Input: part model. Units: mm. Frame: model coordinates. A direction names the side the tool comes from. Give positions to 0.01 mm unless a question says otherwise; leave off trailing zeros. Write each loop counter-clockwise with the first axis right and the second up, starting at its lowest first coordinate (ties: lowest second). Pieces come first, ordered by that corner, then holes.
```python
from build123d import *

# Parameters (mm, degrees)
SKETCH1_W                = 400
SKETCH1_H                = 200
BOSS_EXTRUDE1_DEPTH      = 600
SHELL1_T                 = -10
BOSS_EXTRUDE2_DEPTH      = 25
BOSS_EXTRUDE2_DEPTH_BACK = 10
SKETCH2_W                = 60
SKETCH2_H                = 60
SKETCH3_R                = 7.5
SKETCH3_R_2              = 5
BOSS_EXTRUDE3_DEPTH      = 15
LPATTERN1_COUNT          = 2
LPATTERN1_PITCH          = 330
LPATTERN1_COUNT_DIR2     = 2
LPATTERN1_PITCH_DIR2     = 530
SKETCH4_R                = 15
CUT_EXTRUDE1_DEPTH       = 749.331477355
BOSS_EXTRUDE4_START      = 15
SKETCH5_R                = 25
SKETCH5_R_2              = 15
BOSS_EXTRUDE4_DEPTH      = 15
THICKEN1_START           = 375
THICKEN1_OUTLINE_W       = 31
THICKEN1_OUTLINE_H       = 30
THICKEN1_DEPTH           = 0.5
THICKEN2_START           = 24.5
THICKEN2_OUTLINE_W       = 31
THICKEN2_OUTLINE_H       = 30
THICKEN2_DEPTH           = 0.5
BOSS_EXTRUDE6_REACH      = 737.941
SKETCH7_W                = 380
SKETCH7_H                = 580
SKETCH10_R               = 67.5
CUT_EXTRUDE2_DEPTH       = 60
SKETCH11_R               = 25
BOSS_EXTRUDE7_DEPTH      = 25
BOSS_EXTRUDE8_DEPTH      = 55
SKETCH11_4_R             = 15
CUT_EXTRUDE4_DEPTH       = 20


# Read off the part's stored shape, not the designer's step: Thicken1, Thicken2
with BuildPart() as part:
    # Sketch1 → Boss-Extrude1 (new body)
    with BuildSketch(Plane.XY):
        with Locations((200, 100)):
            Rectangle(SKETCH1_W, SKETCH1_H)
    extrude(amount=BOSS_EXTRUDE1_DEPTH)

    # Shell1
    shell1_openings = [part.faces().sort_by_distance(p)[0] for p in [
        (200, 0, 300),
    ]]
    offset(amount=SHELL1_T, openings=shell1_openings, kind=Kind.INTERSECTION)

    # Sketch2 → Boss-Extrude2 (add, two sides: drawn at the far end of the back side and taken through both)
    with BuildSketch(Plane(origin=(0, 28, 0), x_dir=(1, 0, 0), z_dir=(0, 1, 0)).offset(-BOSS_EXTRUDE2_DEPTH_BACK)):
        with Locations((370, -570)):
            Rectangle(SKETCH2_W, SKETCH2_H)
        with Locations((30, -570)):
            Rectangle(SKETCH2_W, SKETCH2_H)
        with Locations((370, -30)):
            Rectangle(SKETCH2_W, SKETCH2_H)
        with Locations((30, -30)):
            Rectangle(SKETCH2_W, SKETCH2_H)
    extrude(amount=BOSS_EXTRUDE2_DEPTH + BOSS_EXTRUDE2_DEPTH_BACK)

    # Sketch3 → Boss-Extrude3 (add)
    with BuildSketch(Plane(origin=(0, 18, 0), x_dir=(1, 0, 0), z_dir=(0, 1, 0))):
        with Locations(Location((35, -565, 0), (0, 0, 270))):
            Circle(SKETCH3_R)
        with Locations(Location((35, -565, 0), (0, 0, 270))):
            Circle(SKETCH3_R_2, mode=Mode.SUBTRACT)
    boss_extrude3 = extrude(amount=-BOSS_EXTRUDE3_DEPTH)

    # LPattern1: Boss-Extrude3 2 × 2
    with Locations(*[(i * LPATTERN1_PITCH, 0, -j * LPATTERN1_PITCH_DIR2) for i in range(LPATTERN1_COUNT) for j in range(LPATTERN1_COUNT_DIR2) if (i, j) != (0, 0)]):
        add(boss_extrude3)

    # Sketch4 → Cut-Extrude1 (cut, through all)
    with BuildSketch(Plane(origin=(0, 0, 0), x_dir=(0, 0, -1), z_dir=(1, 0, 0))):
        with Locations((-300, 0.8)):
            Circle(SKETCH4_R)
    extrude(amount=CUT_EXTRUDE1_DEPTH, mode=Mode.SUBTRACT)

    # Sketch5 → Boss-Extrude4 (add)
    with BuildSketch(Plane.ZY.offset(-390).offset(BOSS_EXTRUDE4_START)):
        with Locations(Location((300, 0.8, 0), (0, 0, 181.833778))):
            Circle(SKETCH5_R)
        with Locations((300, 0.8)):
            Circle(SKETCH5_R_2, mode=Mode.SUBTRACT)
    boss_extrude4 = extrude(amount=-BOSS_EXTRUDE4_DEPTH)

    # Thicken1 outline → Thicken1 (add)
    with BuildSketch(Plane.YZ.offset(THICKEN1_START)):
        with Locations((0.5, 300)):
            Rectangle(THICKEN1_OUTLINE_W, THICKEN1_OUTLINE_H)
    extrude(amount=THICKEN1_DEPTH)

    # Mirror5: Boss-Extrude4 across plane
    add(boss_extrude4.mirror(Plane(origin=(200, 0, 0), x_dir=(0, 0, 1), z_dir=(1, 0, 0))))

    # Thicken2 outline → Thicken2 (add)
    with BuildSketch(Plane.YZ.offset(THICKEN2_START)):
        with Locations((0.5, 300)):
            Rectangle(THICKEN2_OUTLINE_W, THICKEN2_OUTLINE_H)
    extrude(amount=THICKEN2_DEPTH)

    # Sketch7 → Boss-Extrude6 (add, up to next)
    with BuildSketch(Plane(origin=(0, 53, 0), x_dir=(1, 0, 0), z_dir=(0, 1, 0)), mode=Mode.PRIVATE) as boss_extrude6_sk1:
        with Locations((200, -300)):
            Rectangle(SKETCH7_W, SKETCH7_H)
    boss_extrude6_tool1 = extrude(boss_extrude6_sk1.sketch, amount=BOSS_EXTRUDE6_REACH, mode=Mode.PRIVATE) - part.part
    add(boss_extrude6_tool1.solids().sort_by_distance((200, 53, 300))[0])

    # Sketch10 → Cut-Extrude2 (cut)
    with BuildSketch(Plane(origin=(0, 0, 0), x_dir=(0, 0, -1), z_dir=(1, 0, 0))):
        with Locations((-300, 0.8)):
            Circle(SKETCH10_R)
    cut_extrude2 = extrude(amount=CUT_EXTRUDE2_DEPTH, mode=Mode.SUBTRACT)



with BuildPart() as body_2:
    # Sketch11 → Boss-Extrude7 (new body)
    with BuildSketch(Plane(origin=(60, 0, 0), x_dir=(0, 0, -1), z_dir=(1, 0, 0))):
        with Locations(Location((-300, 0.8, 0), (0, 0, 358.166222))):
            Circle(SKETCH11_R)
    boss_extrude7 = extrude(amount=BOSS_EXTRUDE7_DEPTH)


with BuildPart() as part_1:
    add(part.part)

    add(body_2.part)  # Boss-Extrude8 merges body 2
    # Sketch12 → Boss-Extrude8 (add)
    with BuildSketch(Plane.XZ):
        Polygon((0, 367.495259093), (60, 367.495259093), (60, 325), (60, 274.564639087), (60, 232.504740907), (0, 232.504740907), (0, 222.504740907), (70, 222.504740907), (70, 274.564639087), (70, 325), (70, 377.495259093), (0, 377.495259093), align=None)
    boss_extrude8 = extrude(amount=-BOSS_EXTRUDE8_DEPTH)

    # Sketch11<4> → Cut-Extrude4 (cut)
    with BuildSketch(Plane(origin=(60, 0, 0), x_dir=(0, 0, -1), z_dir=(1, 0, 0))):
        with Locations(Location((-300, 0.8, 0), (0, 0, 183.057225428))):
            Circle(SKETCH11_4_R)
    cut_extrude4 = extrude(amount=CUT_EXTRUDE4_DEPTH, mode=Mode.SUBTRACT)

    # Mirror7: Cut-Extrude2 across plane
    add(cut_extrude2.mirror(Plane(origin=(200, 0, 0), x_dir=(0, 0, 1), z_dir=(1, 0, 0))), mode=Mode.SUBTRACT)

    # Mirror10: Boss-Extrude8 across plane
    add(boss_extrude8.mirror(Plane(origin=(200, 0, 0), x_dir=(0, 0, 1), z_dir=(1, 0, 0))))

    # Mirror14: Boss-Extrude7 across plane
    add(boss_extrude7.mirror(Plane(origin=(200, 0, 0), x_dir=(0, 0, 1), z_dir=(1, 0, 0))))

    # Mirror15: Cut-Extrude4 across plane
    add(cut_extrude4.mirror(Plane(origin=(200, 0, 0), x_dir=(0, 0, 1), z_dir=(1, 0, 0))), mode=Mode.SUBTRACT)


solid = part_1.part
```
Q1. Pin query (flat end, axial travel): pin 1 (12 mm diameter, centred on y = 121.5, z = 341.5, fed in from -X); pin 2 (3 mm diameter, centred on x = 365.5, z = 34, fed in from -Y); pin 3 (2 mm diameter, centred on x = 240, z = 181.5, fed in from -Y); pin 4 (7.5 mm diameter, centred on x = 368, z = 36.5, fed in from -Y). Return the tip coordinate at first contact, or that it passes through.
Q2. Section B-B, the plane x = 306. Return the cut outline in (y, z), then the cut area to 3 significant figures.
Q3. Section C-C, the plane z = 484.5. Return the cut outline in (x, y), then the cut area to 3 significant figures.
Q4. Mould query, pull axis Z, two halves, no side actions, for faces 1 (the flat face through (60, 35, 565)), 2 (the flat face through (197, 101, 0)), 3 (the flat face through (60, 32, 301)). Classes: +Z half, -Z half, draft (parallel to the pull), parting line (faces both ways), or undercut.
Q5. Section A-A, the plane z = 300. Return the cut outline in (x, y), then the cut area to 3 significant figures.
Q6. Material intervals for line 1 along X through (y, z) = (14.75, 565); line 2 along Z through (x, y) = (67.25, 0.8); line 3 along X through (y, z) = (33.5, 205), sorted ascending.
Q7. Access query for faces 4 (the flat face through (10, 26, 138)), 5 (the flat face through (80, 1, 300)), 6 (the cylindrical face through (324.897, -21.737, 289.18)). Directions: +Z, -Z, +X, -X, +Y, -Y. A direction counts if a zero-diameter tool reaches every point of the face in a straight line with its end or side. Return the directions, or none.
Solutions:
1. pin 1: stops at x = 0
1. pin 2: stops at y = 18
1. pin 3: stops at y = 53
1. pin 4: stops at y = 3
2. outline: (0, 0) - (200, 0) - (200, 600) - (0, 600) - (0, 590) - (53, 590) - (53, 10) - (0, 10) - close
2. area: 89,300 mm2
3. outline: (0, 0) - (10, 0) - (10, 53) - (390, 53) - (390, 0) - (400, 0) - (400, 200) - (0, 200) - close
3. area: 59,900 mm2
4. face 1: undercut
4. face 2: -Z half
4. face 3: undercut
5. outline: (0, 68.3) - (60, 68.3) - (60, 15.8) - (80, 15.8) - (80, -14.2) - (60, -14.2) - (60, -24.2) - (85, -24.2) - (85, 25.8) - (70, 25.8) - (70, 53) - (330, 53) - (330, 25.8) - (315, 25.8) - (315, -24.2) - (340, -24.2) - (340, -14.2) - (320, -14.2) - (320, 15.8) - (340, 15.8) - (340, 68.3) - (400, 68.3) - (400, 200) - (0, 200) - close
5. area: 58,800 mm2
6. line 1: x = 0 to 10, 27.5 to 30, 40 to 42.5, 357.5 to 360, 370 to 372.5, 390 to 400
6. line 2: z = 0 to 10, 222.5 to 285, 315 to 377.5, 590 to 600
6. line 3: x = 0 to 10, 390 to 400
7. face 4: -Y
7. face 5: -X
7. face 6: none
